Design review of the part built by this model. Coordinates are the model's own, in mm. A direction names the side the tool comes from. Give positions to 0.01 mm unless a question says otherwise; leave off trailing zeros. Loops run counter-clockwise (first coordinate to the right, second up) from the corner with the lowest first, then second, coordinate; pieces in that order, holes last. Notation, with made-up numbers: (32, 15.25) -> (78, 15.25) arc R10 ccw to (78, 31.25) -> close; hole circle Ø1 at (22, 21.5). An arc over 180 degrees is marked (long way). Use a Markdown table: item, result. Add a question column.
1. Add section C-C (x = 46). State the section outline as (y, z) points, and give its area (3 significant figures).
2. Add section B-B (z = -45.5). State the section outline as (x, y) points.
3. For pin 1 Ø8 at (y, z) = (-39, -24.5) entering from -X; pin 2 Ø2 at (x, y) = (-25.5, -21.5) entering from +Z; pin 3 Ø4.5 at (x, z) = (-46, 0) entering from -Y, all flat-tipped, find the tip position at first contact; note any pin that passes through.
4. For faces 1 (the flat face through (-24, 5, 24)), 2 (the cylindrical face through (-48.794, 2.465, 25.379)), 3 (the flat face through (0, 0, 0)), list the 3-axis set-ups (+Z, -Z, +X, -X, +Y, -Y) from which the entire face can be reached by the end or side of a thin tool; tool diameter is ignored.
5. Draft analysis for pull direction Z (two halves, no side actions). For faces 4 (the flat face through (0, 15, 0)), 5 (the cylindrical face through (-9.76, 10.07, -31)), 6 (the cylindrical face through (0, 2, -48)), state which applies: pulls with the +Z half, pulls with the -Z half, needs draft (parallel to the pull), parting line crosses it, or undercut.
6. To check wall thickness, follow line 1 (X direction, y = 3.6, z = 0); line 2 (X direction, y = -19.5, z = 0); line 3 (Y direction, x = -12, z = -11). State the ranges of each line that lie inside material, in increasing order.
7. Add section D-D (y = -14). State the section outline as (x, z) points.
8. Add section A-A (x = 0). State the section outline as (y, z) points.
```python
from build123d import *

# Parameters (mm, degrees)
SKETCH1_R             = 55
SKETCH1_R_2           = 2
SKETCH1_R_3           = 32.5
BOSS_EXTRUDE1_DEPTH   = 5
SKETCH3_R             = 37.5
SKETCH3_R_2           = 32.5
BOSS_EXTRUDE3_DEPTH   = 50
BOSS_EXTRUDE4_START   = 15
SKETCH1_4_R           = 32.5
BOSS_EXTRUDE4_DEPTH   = 15
CIRPATTERN1_OUTLINE_R = 2
CIRPATTERN1_DEPTH     = 5


# Read off the part's stored shape, not the designer's step: CirPattern1
with BuildPart() as part:
    # Sketch1 → Boss-Extrude1 (new body)
    # profile 1 of 2: a face of its own
    with BuildSketch(Plane(origin=(0, 0, 0), x_dir=(1, 0, 0), z_dir=(0, 1, 0))):
        with Locations(Location((0, 0, 0), (0, 0, 270))):
            Circle(SKETCH1_R)
        with Locations(Location((0, 46, 0), (0, 0, 270))):
            Circle(SKETCH1_R_2, mode=Mode.SUBTRACT)
        Circle(SKETCH1_R_3, mode=Mode.SUBTRACT)
    # profile 2 of 2: a face of its own
    with BuildSketch(Plane(origin=(0, 0, 0), x_dir=(1, 0, 0), z_dir=(0, 1, 0))):
        Circle(SKETCH1_R_3)
    extrude(amount=BOSS_EXTRUDE1_DEPTH)

    # Sketch3 → Boss-Extrude3 (add)
    with BuildSketch(Plane.XZ):
        with Locations(Location((0, 0, 0), (0, 0, 90))):
            Circle(SKETCH3_R)
        with Locations(Location((0, 0, 0), (0, 0, 270))):
            Circle(SKETCH3_R_2, mode=Mode.SUBTRACT)
    extrude(amount=BOSS_EXTRUDE3_DEPTH)

    # Sketch1<4> → Boss-Extrude4 (add)
    with BuildSketch(Plane(origin=(0, 0, 0), x_dir=(1, 0, 0), z_dir=(0, 1, 0)).offset(BOSS_EXTRUDE4_START)):
        with Locations(Location((0, 0, 0), (0, 0, 90))):
            Circle(SKETCH1_4_R)
    extrude(amount=-BOSS_EXTRUDE4_DEPTH)

    # CirPattern1 outline → CirPattern1 (cut)
    with BuildSketch(Plane(origin=(0, 0, 0), x_dir=(1, 0, 0), z_dir=(0, 1, 0))):
        with Locations((46, 0)):
            Circle(CIRPATTERN1_OUTLINE_R)
        with Locations((0, -46)):
            Circle(CIRPATTERN1_OUTLINE_R)
        with Locations((-46, 0)):
            Circle(CIRPATTERN1_OUTLINE_R)
    extrude(amount=CIRPATTERN1_DEPTH, mode=Mode.SUBTRACT)


solid = part.part
```
Taken from the geometry:
| question | item | result |
|---|---|---|
| 1 | outline | (0, -30.15) -> (5, -30.15) -> (5, -2) -> (0, -2) -> close; (0, 2) -> (5, 2) -> (5, 30.15) -> (0, 30.15) -> close |
| 1 | area | 281 mm^2 |
| 2 | outline | (-30.9, 0) -> (-1.94, 0) -> (-1.94, 5) -> (-30.9, 5) -> close; (1.94, 0) -> (30.9, 0) -> (30.9, 5) -> (1.94, 5) -> close |
| 3 | pin 1 | stops at x = -31.4 |
| 3 | pin 2 | stops at z = 28.39 |
| 3 | pin 3 | stops at y = 0 |
| 4 | face 1 | +Y |
| 4 | face 2 | +Y, -Y |
| 4 | face 3 | -Y |
| 5 | face 4 | needs draft |
| 5 | face 5 | parting line crosses it |
| 5 | face 6 | undercut |
| 6 | line 1 | x = -55 to -48, -44 to 44, 48 to 55 |
| 6 | line 2 | x = -37.5 to -32.5, 32.5 to 37.5 |
| 6 | line 3 | y = 0 to 15 |
| 7 | outline | circle Ø75 at (0, 0); hole circle Ø65 at (0, 0) |
| 8 | outline | (-50, -37.5) -> (0, -37.5) -> (0, -44) -> (5, -44) -> (5, -32.5) -> (15, -32.5) -> (15, 32.5) -> (5, 32.5) -> (5, 44) -> (0, 44) -> (0, 37.5) -> (-50, 37.5) -> (-50, 32.5) -> (0, 32.5) -> (0, -32.5) -> (-50, -32.5) -> close; (0, -55) -> (5, -55) -> (5, -48) -> (0, -48) -> close; (0, 48) -> (5, 48) -> (5, 55) -> (0, 55) -> close |
